Autodesk Inventor part; units mm, degrees
ref_plane "YZ Plane" through (0, 0, 0) normal (1, 0, 0) x (0, 1, 0)
ref_plane "XZ Plane" through (0, 0, 0) normal (0, 1, 0) x (-1, 0, 0)
ref_plane "XY Plane" through (0, 0, 0) normal (0, 0, 1) x (1, 0, 0)
sketch "body" plane through (0, 0, 0) normal (0, 0, 1) x (1, 0, 0)
  line L0 (-19.15, -21.15) -> (19.15, -21.15)
  line L1 (21.15, -19.15) -> (21.15, 19.15)
  line L2 (19.15, 21.15) -> (-19.15, 21.15)
  line L3 (-21.15, 19.15) -> (-21.15, -19.15)
  line L4 (-21.15, -21.15) -> (21.15, 21.15) construction
  line L5 (21.15, -21.15) -> (-21.15, 21.15) construction
  line L6 (-19.15, -21.15) -> (-21.15, -19.15)
  line L7 (-21.15, 19.15) -> (-19.15, 21.15)
  line L8 (21.15, 19.15) -> (19.15, 21.15)
  line L9 (19.15, -21.15) -> (21.15, -19.15)
  circle A0 centre (-15.5, 15.5) radius 1.5
  circle A1 centre (15.5, 15.5) radius 1.5
  circle A2 centre (15.5, -15.5) radius 1.5
  circle A3 centre (-15.5, -15.5) radius 1.5
  point P0 (0, 0)
  dimension "d5" = 42.3
  dimension "d6" = 42.3
  dimension "d7" = 2
  dimension "d8" = 2
  dimension "d9" = 2
  dimension "d10" = 2
  dimension "d11" = 2
  dimension "d12" = 2
  dimension "d13" = 2
  dimension "d14" = 2
  dimension "d15" = 3
  dimension "d16" = 3
  dimension "d17" = 3
  dimension "d18" = 3
sketch "Sketch6" plane through (0, 0, 0) normal (0, 0, 1) x (1, 0, 0)
  circle A0 centre (0, 0) radius 2.5
  dimension "d19" = 5
extrude "Extrusion1" add sketch "body" along normal blind 34
extrude "Extrusion2" add sketch "Sketch6" against normal blind 24
equation "\"d8\" = d7"
equation "\"d10\" = d9"
equation "\"d11\" = d9"
equation "\"d12\" = d11"
equation "\"d13\" = d9"
equation "\"d14\" = d13"
properties part number "motor"
Can you work these out from the model? Positions are in its coordinate system, mm. A direction names the side the tool comes from. Coordinates: 2 decimals unless noted, no trailing zeros. Write each loop counter-clockwise with the first axis right and the second up, starting at its lowest first coordinate (ties: lowest second). Pieces come first, ordered by that corner, then holes. Notation, with made-up numbers: (82.5, -16) - (87.5, -16) arc R20 ccw to (87.5, 18) - close; hole circle Ø7 at (73.25, 77.25). An arc over 180 degrees is marked (long way). Return JSON: item names as keys, results as strings.
Q1. If we section it at D-D (y = 0): Please give me the cut outline in (x, z), then the cut area to 3 significant figures.
Computed values:
{"outline": "(-21.15, 0) - (-2.5, 0) - (-2.5, -24) - (2.5, -24) - (2.5, 0) - (21.15, 0) - (21.15, 34) - (-21.15, 34) - close", "area": "1,560 mm2"}
Q2. Thinking about a two-plate mould opening in Y: for faces 3 (the flat face through (0, -21.15, 17)), 4 (the cylindrical face through (-17, 15.43, 16.76)), 5 (the flat face through (-20.2, 20.1, 16.8)), which applies, +Y half, -Y half, draft (parallel to the pull), parting line (faces both ways), or undercut?
Computed values:
{"face 3": "-Y half", "face 4": "undercut", "face 5": "+Y half"}
Q3. If we section it at C-C (z = 18.5): Please give me the cut outline in (x, y), then the cut area to 3 significant figures.
Computed values:
{"outline": "(-21.15, -19.15) - (-19.15, -21.15) - (19.15, -21.15) - (21.15, -19.15) - (21.15, 19.15) - (19.15, 21.15) - (-19.15, 21.15) - (-21.15, 19.15) - close; hole circle Ø3 at (-15.5, -15.5); hole circle Ø3 at (-15.5, 15.5); hole circle Ø3 at (15.5, -15.5); hole circle Ø3 at (15.5, 15.5)", "area": "1,750 mm2"}
Q4. If we section it at A-A (y = 15.5): Please give me the cut outline in (x, z).
Computed values:
{"outline": "(-21.15, 0) - (-17, 0) - (-17, 34) - (-21.15, 34) - close; (-14, 0) - (14, 0) - (14, 34) - (-14, 34) - close; (17, 0) - (21.15, 0) - (21.15, 34) - (17, 34) - close"}
Q5. Please list where these lines run through material, in increasing order: L1, parallel to Y at x = -15.5, z = 19; L2, parallel to Z at x = 8, y = 2.5; L3, parallel to X at y = 14.5, z = 20. Write a range as from..to.
Computed values:
{"L1": "y = -21.15..-17, -14..14, 17..21.15", "L2": "z = 0..34", "L3": "x = -21.15..-16.62, -14.38..14.38, 16.62..21.15"}
Q6. I'm going to push a flat-ended pin straight in: pin 1 Ø1 at (x, y) = (-11, -7.5) entering from -Z. Where does the tip first touch, or does it pass through?
Computed values:
{"pin 1": "stops at z = 0"}
Q7. On a 3-axis mill with a long thin cutter (end or side, diameter ignored), from which of +Z, -Z, +X, -X, +Y, -Y can I reach the whole of each face in a straight line? I mean faces 1 (the cylindrical face through (-0.54, -2.44, -11.83)), 2 (the flat face through (-20.1, -20.2, 16.8)). Say none if no direction works.
Computed values:
{"face 1": "-Z", "face 2": "+Z, -Z, -X, -Y"}
